```python
from build123d import *

# Parameters (mm, degrees)
SKETCH1_W                  = 109.5
SKETCH1_H                  = 82.5
BOSS_EXTRUDE1_DEPTH        = 2
F_3_5_3_5_DIAMETER_HOLE1_D = 3.5
F_2_6_2_6_DIAMETER_HOLE1_D = 2.6
SKETCH9_R                  = 3
CUT_EXTRUDE1_DEPTH         = 1
F_2_2_2_2_DIAMETER_HOLE1_D = 2.2
FILLET1_R                  = 1
FILLET2_R                  = 3


with BuildPart() as part:
    # Sketch1 → Boss-Extrude1 (new body)
    with BuildSketch(Plane.XY):
        with Locations((0, -41.75)):
            Rectangle(SKETCH1_W, SKETCH1_H)
        with BuildLine():
            Line((28.75, -9.25), (28.75, -13.6))
            ThreePointArc((28.75, -13.6), (29.628679656, -15.721320344), (31.75, -16.6))
            Line((31.75, -16.6), (41.75, -16.6))
            ThreePointArc((41.75, -16.6), (43.871320344, -17.478679656), (44.75, -19.6))
            Line((44.75, -19.6), (44.75, -31.75))
            Line((44.75, -31.75), (48.75, -31.75))
            Line((48.75, -31.75), (48.75, -41.75))
            Line((48.75, -41.75), (48.75, -51.75))
            Line((48.75, -51.75), (44.75, -51.75))
            Line((44.75, -51.75), (44.75, -74.25))
            ThreePointArc((44.75, -74.25), (43.871320344, -76.371320344), (41.75, -77.25))
            Line((41.75, -77.25), (-41.75, -77.25))
            ThreePointArc((-41.75, -77.25), (-43.871320344, -76.371320344), (-44.75, -74.25))
            Line((-44.75, -74.25), (-44.75, -51.75))
            Line((-44.75, -51.75), (-48.75, -51.75))
            Line((-48.75, -51.75), (-48.75, -31.75))
            Line((-48.75, -31.75), (-44.75, -31.75))
            Line((-44.75, -31.75), (-44.75, -9.25))
            ThreePointArc((-44.75, -9.25), (-43.871320344, -7.128679656), (-41.75, -6.25))
            Line((-41.75, -6.25), (25.75, -6.25))
            ThreePointArc((25.75, -6.25), (27.871320344, -7.128679656), (28.75, -9.25))
        make_face(mode=Mode.SUBTRACT)
    extrude(amount=BOSS_EXTRUDE1_DEPTH)

    # Ø3.5 (3.5) Diameter Hole1 (through all)
    with Locations(Plane.XY.offset(2)):
        with Locations((-48.25, -3.75), (-48.25, -79.75), (48.25, -79.75), (48.25, -3.75)):
            Hole(F_3_5_3_5_DIAMETER_HOLE1_D / 2)

    # Sketch5 → CSK for M2.5 Flat Countersunk Head Screw1 (revolve, cut)
    with BuildSketch(Plane(origin=(33.65, -12.1, 2), x_dir=(0, -1, 0), z_dir=(1, 0, 0))):
        Polygon((0, 0), (0, 2), (1.35, 2), (1.35, 1.5), (2.85, 0), align=None)
    revolve(axis=Axis((33.65, -12.1, 8.35), (0, 0, -1)), mode=Mode.SUBTRACT)

    # Ø2.6 (2.6) Diameter Hole1 (through all)
    with Locations(Plane.XY.offset(2)):
        with Locations((33.65, -2.57)):
            Hole(F_2_6_2_6_DIAMETER_HOLE1_D / 2)

    # Sketch9 → Cut-Extrude1 (cut)
    with BuildSketch(Plane.XY.offset(2)):
        with Locations((-48.25, -3.75)):
            Circle(SKETCH9_R)
        with Locations((48.25, -3.75)):
            Circle(SKETCH9_R)
        with Locations((48.25, -79.75)):
            Circle(SKETCH9_R)
        with Locations((-48.25, -79.75)):
            Circle(SKETCH9_R)
    extrude(amount=-CUT_EXTRUDE1_DEPTH, mode=Mode.SUBTRACT)

    # Ø2.2 (2.2) Diameter Hole1 (through all)
    with Locations(Plane.XY.offset(2)):
        with Locations((-24.75, -3.25), (24.75, -3.25), (-24.75, -80.25), (24.75, -80.25)):
            Hole(F_2_2_2_2_DIAMETER_HOLE1_D / 2)

    # Fillet1
    fillet1_edges = [part.edges().sort_by_distance(p)[0] for p in [
        (-44.75, -31.75, 1),
        (-44.75, -51.75, 1),
        (44.75, -51.75, 1),
        (44.75, -31.75, 1),
    ]]
    fillet(fillet1_edges, radius=FILLET1_R)

    # Fillet2
    fillet2_edges = [part.edges().sort_by_distance(p)[0] for p in [
        (48.75, -31.75, 1),
        (48.75, -51.75, 1),
        (-48.75, -51.75, 1),
        (-48.75, -31.75, 1),
    ]]
    fillet(fillet2_edges, radius=FILLET2_R - 0.0001)  # a hair under: the kernel refuses the full size


solid = part.part
```
The model under review builds one solid part; all positions refer to its coordinate system, in mm. A direction names the side the tool comes from. Coordinates: 2 decimals unless noted, no trailing zeros. Write each loop counter-clockwise with the first axis right and the second up, starting at its lowest first coordinate (ties: lowest second). Pieces come first, ordered by that corner, then holes. Notation, with made-up numbers: (19.5, -12) -> (28.5, -12) arc R4 ccw to (28.5, -8) -> close; hole circle Ø10 at (-3, 69). An arc over 180 degrees is marked (long way). One line per item, written item: value. Start each with the question number.
Q1. Add section A-A, the plane y = -66.5. Give the boundary of the cut face in (x, z), then the cut area to 3 significant figures.
Q2. To check wall thickness, follow probe 1 along Y at (x, z) = (-24.75, 1.15); probe 2 along Y at (x, z) = (33.5, 0.35); probe 3 along X at (y, z) = (-29, 1.4). State the ranges of each line that lie inside material, in increasing order.
Q3. The part is to be moulded in two halves that separate along Y. For faces 1 (the face through (-48.9, -82.68, 1.51)), 2 (the face through (0, -5, 2)), 3 (the face through (29.61, -15.7, 0.99)), say which applies: +Y half, -Y half, draft (parallel to the pull), parting line (faces both ways), or undercut.
Q4. Add section C-C, the plane z = 1.4. Count the separate pieces of the cut face and the enclosed holes in it, then the cut area to 3 significant figures.
Q5. Clearance check with a flat-ended pin moving along its axis: P1, Ø4.5, axis at x = 33.65, y = -12.1, coming from the +Z side. State where the tip first meets the part, or that it passes through.
Q6. Add section B-B, the plane x = 19. Give the boundary of the cut face in (y, z), then the cut area to 3 significant figures.
Q7. For faces 4 (the face through (43.89, -76.35, 0.99)), 5 (the face through (45.869, -81.575, 1.507)), list the 3-axis set-ups (+Z, -Z, +X, -X, +Y, -Y) from which the entire face can be reached by the end or side of a thin tool; tool diameter is ignored.
Response:
1. outline: (-54.75, 0) -> (-44.75, 0) -> (-44.75, 2) -> (-54.75, 2) -> close; (44.75, 0) -> (54.75, 0) -> (54.75, 2) -> (44.75, 2) -> close
1. area: 40.0 mm²
2. probe 1: -83 to -81.35, -79.15 to -77.25, -6.25 to -4.35, -2.15 to -0.5
2. probe 2: -83 to -77.25, -16.6 to -13.44, -10.76 to -3.86, -1.28 to -0.5
2. probe 3: -54.75 to -44.75, 44.75 to 54.75
3. face 1: undercut
3. face 2: draft
3. face 3: undercut
4. separate pieces: 1
4. enclosed holes: 11
4. area: 2,550 mm²
5. P1: z = 1.4
6. outline: (-83, 0) -> (-77.25, 0) -> (-77.25, 2) -> (-83, 2) -> close; (-6.25, 0) -> (-0.5, 0) -> (-0.5, 2) -> (-6.25, 2) -> close
6. area: 23.0 mm²
7. face 4: +Z, -Z
7. face 5: +Z
